For this review, take the finished solid that the model builds, in its own axes (mm). Coordinates: 2 decimals unless noted, no trailing zeros. Write each loop counter-clockwise with the first axis right and the second up, starting at its lowest first coordinate (ties: lowest second). Pieces come first, ordered by that corner, then holes. Notation, with made-up numbers: (-28, -19) -> (23, -19) arc R33 cw to (23, 17) -> close; hole circle Ø6 at (-10, 43). An arc over 180 degrees is marked (long way). One line per item, written item: value. Start each with the question number.
1) For probe 1 along Y at (x, z) = (8.25, 203) (3 decimals); probe 2 along Z at (x, y) = (10.95, -12.7); probe 3 along X at (y, z) = (-0.5, 79) (3 decimals), list the stretches that pass through material, from the lowest coordinate up. Write a range as from..to.
2) Add section B-B (y = 1). State the section outline as (x, z) points (3 decimals).
3) For pin 1 Ø4 at (x, z) = (0, 6.35) entering from +Y; pin 2 Ø4 at (y, z) = (12.7, 151.003) entering from +X (3 decimals); pin 3 Ø7.5 at (x, z) = (0, 57.15) entering from +Y, all flat-tipped, find the tip position at first contact; note any pin that passes through.
4) Add section A-A (z = 353.5). State the section outline as (x, y) points (3 decimals), and give its area (3 significant figures).
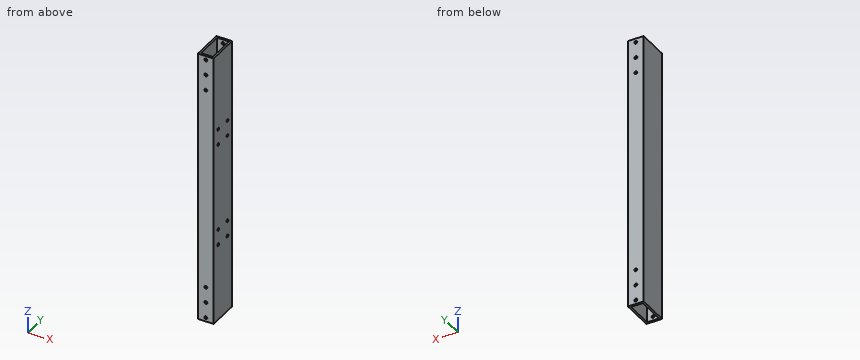
from build123d import *

# Parameters (mm, degrees)
SKETCH1_W           = 25.4
SKETCH1_H           = 50.8
BOSS_EXTRUDE1_DEPTH = 444.5
SHELL1_T            = -3.175
SKETCH2_R           = 2.38125
CUT_EXTRUDE1_DEPTH  = 448.573658742
SKETCH3_R           = 2.38125
CUT_EXTRUDE2_DEPTH  = 6.35


with BuildPart() as part:
    # Sketch1 → Boss-Extrude1 (new body)
    with BuildSketch(Plane.XY):
        Rectangle(SKETCH1_W, SKETCH1_H)
    extrude(amount=BOSS_EXTRUDE1_DEPTH)

    # Shell1
    shell1_openings = [part.faces().sort_by_distance(p)[0] for p in [
        (0, 0, 444.5),
        (0, 0, 0),
    ]]
    offset(amount=SHELL1_T, openings=shell1_openings, kind=Kind.INTERSECTION)

    # Sketch2 → Cut-Extrude1 (cut, through all)
    with BuildSketch(Plane(origin=(0, 25.4, 0), x_dir=(1, 0, 0), z_dir=(0, 1, 0))):
        with Locations(Location((0, -6.35, 0), (0, 0, 270))):
            Circle(SKETCH2_R)
        with Locations(Location((0, -31.75, 0), (0, 0, 270))):
            Circle(SKETCH2_R)
        with Locations(Location((0, -57.15, 0), (0, 0, 270))):
            Circle(SKETCH2_R)
        with Locations(Location((0, -387.35, 0), (0, 0, 270))):
            Circle(SKETCH2_R)
        with Locations(Location((0, -412.75, 0), (0, 0, 270))):
            Circle(SKETCH2_R)
        with Locations(Location((0, -438.15, 0), (0, 0, 270))):
            Circle(SKETCH2_R)
    extrude(amount=-CUT_EXTRUDE1_DEPTH, mode=Mode.SUBTRACT)

    # Sketch3 → Cut-Extrude2 (cut)
    with BuildSketch(Plane(origin=(12.7, 0, 0), x_dir=(0, 0, -1), z_dir=(1, 0, 0))):
        with Locations(Location((-125.603, -12.7, 0), (0, 0, 90))):
            Circle(SKETCH3_R)
        with Locations(Location((-125.603, 12.7, 0), (0, 0, 90))):
            Circle(SKETCH3_R)
        with Locations(Location((-151.003, 12.7, 0), (0, 0, 90))):
            Circle(SKETCH3_R)
        with Locations(Location((-151.003, -12.7, 0), (0, 0, 90))):
            Circle(SKETCH3_R)
        with Locations(Location((-293.497, -12.7, 0), (0, 0, 270))):
            Circle(SKETCH3_R)
        with Locations(Location((-293.497, 12.7, 0), (0, 0, 270))):
            Circle(SKETCH3_R)
        with Locations(Location((-318.897, 12.7, 0), (0, 0, 270))):
            Circle(SKETCH3_R)
        with Locations(Location((-318.897, -12.7, 0), (0, 0, 270))):
            Circle(SKETCH3_R)
    extrude(amount=-CUT_EXTRUDE2_DEPTH, mode=Mode.SUBTRACT)


solid = part.part
Numbers:
1. probe 1: -25.4..-22.225, 22.225..25.4
1. probe 2: 0..123.22, 127.98..148.62, 153.38..291.12, 295.88..316.52, 321.28..444.5
1. probe 3: -12.7..-9.525, 9.525..12.7
2. outline: (-12.7, 0) -> (-9.525, 0) -> (-9.525, 444.5) -> (-12.7, 444.5) -> close; (9.525, 0) -> (12.7, 0) -> (12.7, 444.5) -> (9.525, 444.5) -> close
3. pin 1: through
3. pin 2: x = -9.525
3. pin 3: y = 25.4
4. outline: (-12.7, -25.4) -> (12.7, -25.4) -> (12.7, 25.4) -> (-12.7, 25.4) -> close; hole (-9.525, -22.225) -> (9.525, -22.225) -> (9.525, 22.225) -> (-9.525, 22.225) -> close
4. area: 444 mm²
